```python
from build123d import *

# Parameters (mm, degrees)
SKETCH_1_W               = 23
SKETCH_1_H               = 27.6
SKETCH_1_W_2             = 4.5
SKETCH_1_H_2             = 1
EXTRUDE_1_DEPTH          = 6
SKETCH_2_R               = 3
EXTRUDE_2_DEPTH          = 5
CUT_EXTRUDE_1_DEPTH      = 28.541967976
CUT_EXTRUDE_1_DEPTH_BACK = 28.541967976
SKETCH_3_R               = 1
FILLET_1_R               = 2


with BuildPart() as part:
    # Эскиз1 → Бобышка-Вытянуть1 (new, symmetric)
    with BuildSketch(Plane.XY):
        Rectangle(SKETCH_1_W, SKETCH_1_H)
        with Locations((-13.75, 7.3)):
            Rectangle(SKETCH_1_W_2, SKETCH_1_H_2)
        with Locations((13.75, 7.3)):
            Rectangle(SKETCH_1_W_2, SKETCH_1_H_2)
    extrude(amount=EXTRUDE_1_DEPTH, both=True)

    # Эскиз2 → Бобышка-Вытянуть2 (add)
    with BuildSketch(Plane(origin=(0, 13.8, 0), x_dir=(1, 0, 0), z_dir=(0, 1, 0))):
        with Locations(Location((-7.5, 0, 0), (0, 0, 270))):
            Circle(SKETCH_2_R)
    extrude(amount=EXTRUDE_2_DEPTH)

    # Эскиз3 → Вырез-Вытянуть1 (cut, two sides: drawn at the far end of the back side and taken through both)
    with BuildSketch(Plane(origin=(0, 7.8, 0), x_dir=(1, 0, 0), z_dir=(0, 1, 0)).offset(-CUT_EXTRUDE_1_DEPTH_BACK)):
        with Locations(Location((-13.75, 3.5, 0), (0, 0, 180))):
            Circle(SKETCH_3_R)
        with Locations(Location((-13.75, -3.5, 0), (0, 0, 180))):
            Circle(SKETCH_3_R)
        with Locations(Location((13.75, -3.5, 0), (0, 0, 180))):
            Circle(SKETCH_3_R)
        with Locations(Location((13.75, 3.5, 0), (0, 0, 180))):
            Circle(SKETCH_3_R)
    extrude(amount=CUT_EXTRUDE_1_DEPTH + CUT_EXTRUDE_1_DEPTH_BACK, mode=Mode.SUBTRACT)

    # Скругление1
    fillet_1_edges = [part.edges().sort_by_distance(p)[0] for p in [
        (-16, 7.3, -6),
        (16, 7.3, -6),
        (16, 7.3, 6),
        (-16, 7.3, 6),
    ]]
    fillet(fillet_1_edges, radius=FILLET_1_R)


solid = part.part
```
The listing builds one solid part. Answer for the finished solid, in the listing's coordinates (mm). A direction names the side the tool comes from. Coordinates: 2 decimals unless noted, no trailing zeros. Write each loop counter-clockwise with the first axis right and the second up, starting at its lowest first coordinate (ties: lowest second). Pieces come first, ordered by that corner, then holes. Notation, with made-up numbers: (49.5, 54) - (93.5, 54) arc R33 cw to (93.5, 82) - close; hole circle Ø11 at (56.25, 83). An arc over 180 degrees is marked (long way). Return JSON: item names as keys, results as strings. Group by question number.
Q1. The part is cut by section D-D on y = 10. Write down the section's boundary in (x, z), and give its area (3 significant figures).
Q2. The part is cut by section C-C on x = -10. Write down the section's boundary in (y, z), and give its area (3 significant figures).
Q3. For a pull along X with two mould halves and no side action, classify faces 1 (the flat face through (0, 0, 6)), 2 (the cylindrical face through (-14.704, 7.293, -3.2)), 3 (the cylindrical face through (15.4, 7.31, 5.43)), 4 (the cylindrical face through (-15.4, 7.31, 5.43)) as +X half, -X half, draft (parallel to the pull), parting line (faces both ways), or undercut.
Q4. Which of the six approach directions +Z, -Z, +X, -X, +Y, -Y give full straight-line access (tool end or side, diameter ignored) to faces 5 (the flat face through (-14, 6.8, 0)), 6 (the flat face through (14, 7.8, 0)), 7 (the flat face through (-11.5, 11, 0))?
Q5. The part is cut by section B-B on z = 0. Write down the section's boundary in (x, y), and give its area (3 significant figures).
Q6. The part is cut by section A-A on z = 3.5. Write down the section's boundary in (x, y), and give its area (3 significant figures).
Q7. Find the intervals of material crossed by line 1 along X through (y, z) = (7.4, -3.5); line 2 along Z through (x, y) = (-13.75, 7); line 3 along Y through (x, z) = (6, -3.75), in increasing order. Write a range as [from, to].
Q8. Flat-ended cylindrical pins translate along their axes: pin 1 Ø6 at (x, z) = (8, -2.5) entering from +Y; pin 2 Ø1.3 at (x, z) = (-14, -1.5) entering from +Y; pin 3 Ø1.8 at (y, z) = (11.5, -1) entering from -X. Find the tip coordinate at first contact, or state that the pin passes through.
Evaluation:
{
 "1": {"outline": "(-11.5, -6) - (11.5, -6) - (11.5, 6) - (-11.5, 6) - close", "area": "276 mm2"},
 "2": {"outline": "(-13.8, -6) - (13.8, -6) - (13.8, -1.66) - (18.8, -1.66) - (18.8, 1.66) - (13.8, 1.66) - (13.8, 6) - (-13.8, 6) - close", "area": "348 mm2"},
 "3": {"face 1": "draft", "face 2": "undercut", "face 3": "+X half", "face 4": "-X half"},
 "4": {"face 5": "+Z, -Z, -X, -Y", "face 6": "+Z, -Z, +X, +Y", "face 7": "+Z, -Z, -X, +Y"},
 "5": {"outline": "(-16, 6.8) - (-11.5, 6.8) - (-11.5, -13.8) - (11.5, -13.8) - (11.5, 6.8) - (16, 6.8) - (16, 7.8) - (11.5, 7.8) - (11.5, 13.8) - (-4.5, 13.8) - (-4.5, 18.8) - (-10.5, 18.8) - (-10.5, 13.8) - (-11.5, 13.8) - (-11.5, 7.8) - (-16, 7.8) - close", "area": "674 mm2"},
 "6": {"outline": "(-16, 6.8) - (-14.75, 6.8) - (-14.75, 7.8) - (-16, 7.8) - close; (-12.75, 6.8) - (-11.5, 6.8) - (-11.5, -13.8) - (11.5, -13.8) - (11.5, 6.8) - (12.75, 6.8) - (12.75, 7.8) - (11.5, 7.8) - (11.5, 13.8) - (-11.5, 13.8) - (-11.5, 7.8) - (-12.75, 7.8) - close; (14.75, 6.8) - (16, 6.8) - (16, 7.8) - (14.75, 7.8) - close", "area": "640 mm2"},
 "7": {"line 1": "x = [-16, -14.75], [-12.75, 12.75], [14.75, 16]", "line 2": "z = [-6, -4.5], [-2.5, 2.5], [4.5, 6]", "line 3": "y = [-13.8, 13.8]"},
 "8": {"pin 1": "stops at y = 13.8", "pin 2": "stops at y = 7.8", "pin 3": "stops at x = -11.5"}
}
